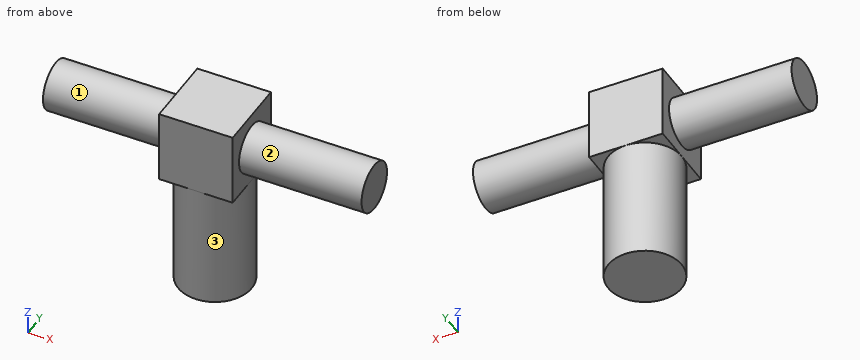
from build123d import *

# Parameters (mm, degrees)
F0_W     = 30
F0_H     = 30
F1_DEPTH = 30
F2_R     = 15
F3_DEPTH = 50
F4_R     = 10
F5_DEPTH = 50
F6_R     = 10
F7_DEPTH = 50


with BuildPart() as f1:
    # F0 (on Top) → F1 (new body)
    with BuildSketch(Plane.XY):
        Rectangle(F0_W, F0_H)
    extrude(amount=F1_DEPTH)

    # F2 (on face) → F3 (join)
    with BuildSketch(Plane(origin=(0, 0, 0), x_dir=(1, 0, 0), z_dir=(0, 0, -1))):
        Circle(F2_R)
    extrude(amount=F3_DEPTH)

    # F4 (on face) → F5 (join)
    with BuildSketch(Plane.YZ.offset(15)):
        with Locations((0, 15)):
            Circle(F4_R)
    extrude(amount=F5_DEPTH)

    # F6 (on face) → F7 (join)
    with BuildSketch(Plane(origin=(-15, 0, 0), x_dir=(0, -1, 0), z_dir=(-1, 0, 0))):
        with Locations((0, 15)):
            Circle(F6_R)
    extrude(amount=F7_DEPTH)


solid = f1.part
Model file for the job. Use its own axes, mm. Face numbers are marked on the shaded views. A direction names the side the tool comes from. Round coordinates to 2 decimals unless told otherwise and drop trailing zeros. Loops run counter-clockwise (first coordinate to the right, second up) from the corner with the lowest first, then second, coordinate; pieces in that order, holes last. Notation, with made-up numbers: M -9,69.5 L 7,69.5 A29 ccw 7,91.5 Z; hole C 60,80 d8. An arc over 180 degrees is marked long. One line per question, with ' | ' between items.
1) Drill centre lines: line 1 along X through (y, z) = (-7.5, 4.5); line 2 along X through (y, z) = (-6.5, -27.5); line 3 along Z through (x, y) = (16, 8.25). Where is each one in solid material? Low to high.
Solved:
line 1: x = -15 to 15 | line 2: x = -13.52 to 13.52 | line 3: z = 9.35 to 20.65
2) Band-saw the part on B-B (y = -12.25). Give the cut face in (x, z).
Solved:
outline: M -15,0 L -8.66,0 L -8.66,-50 L 8.66,-50 L 8.66,0 L 15,0 L 15,30 L -15,30 Z
3) Band-saw the part on D-D (y = 11.5). Give the cut face in (x, z), then the cut area to 3 significant figures.
Solved:
outline: M -15,0 L -9.63,0 L -9.63,-50 L 9.63,-50 L 9.63,0 L 15,0 L 15,30 L -15,30 Z | area: 1,860 mm²
4) 3-axis set-ups, long thin cutter, end or side, ignore diameter. For the marked faces 1, 2 and 3: which of +Z, -Z, +X, -X, +Y, -Y reach the whole face in a straight line?
Solved:
face 1: -X | face 2: +X | face 3: -Z
5) Band-saw the part on A-A (z = 15). Give the cut face in (x, y), then the cut area to 3 significant figures.
Solved:
outline: M -65,-10 L -15,-10 L -15,-15 L 15,-15 L 15,-10 L 65,-10 L 65,10 L 15,10 L 15,15 L -15,15 L -15,10 L -65,10 Z | area: 2,900 mm²
6) Band-saw the part on C-C (x = 36.5). Give the cut face in (y, z).
Solved:
outline: C 0,15 d20
7) Flat gauge pins, fed straight in: pin 1 (2 mm diameter, centred on y = -5, z = -27, fed in from +X); pin 2 (3 mm diameter, centred on y = -7, z = -13.5, fed in from +X); pin 3 (8 mm diameter, centred on x = -42.5, y = 3, fed in from -Z). Where does each tip first touch, or does it go through?
Solved:
pin 1: stops at x = 14.46 | pin 2: stops at x = 13.96 | pin 3: stops at z = 5
